Model file for the job. Use its own axes, mm. A direction names the side the tool comes from. Round coordinates to 2 decimals unless told otherwise and drop trailing zeros. Order: outer loops, then holes, each group sorted by start corner. A loop starts at its lowest first (then second) coordinate and runs counter-clockwise, first axis right, second up. Notation, with made-up numbers: (37, -31.75) -> (46, -31.75) arc R21 cw to (46, -26.75) -> close; hole circle Ø7 at (-35.75, -30.5). An arc over 180 degrees is marked (long way). Put each result on its own line as item: value. Start each with the question number.
Q1. Cut at B-B, the plane y = 91.5. List the corners of the cut face in (x, z).
Q2. Flat gauge pin, fed straight in: P1, Ø3, axis at y = 124, z = 3, coming from the +X side. Where does the tip first touch, or does it go through?
Q3. Probe L1, parallel to Y at x = 273, z = 3.9; L2, parallel to X at y = 174, z = 2.9; L3, parallel to X at y = 10, z = 4.1. List the from-to ranges inside material, lowest first.
Q4. Pull direction Y, two halves, no side cores. Call faces 1 (the face through (0, 99, 3)), 2 (the face through (25, 99, 3)), 3 (the face through (148, 0, 3)): released by +Y, released by -Y, zero draft, split by the parting line, or undercut.
Q5. 3-axis set-ups, long thin cutter, end or side, ignore diameter. For faces 4 (the face through (226, 40, 3)), 5 (the face through (115, 101, 6)), 6 (the face through (30, 99, 3)): which of +Z, -Z, +X, -X, +Y, -Y reach the whole face in a straight line?
Q6. Cut at C-C, the plane z = 3.15. State how many separate pieces and enclosed holes the cut face has, and give its area (3 significant figures).
Q7. Cut at A-A, the plane x = 217.5. List the corners of the cut face in (y, z).
from build123d import *

# Parameters (mm, degrees)
SKETCH1_W                       = 300
SKETCH1_H                       = 200
BOSS_EXTRUDE1_DEPTH             = 6
SKETCH2_W                       = 145
SKETCH2_H                       = 120
CUT_EXTRUDE1_DEPTH              = 6
SKETCH3_W                       = 5
SKETCH3_H                       = 160
CUT_EXTRUDE2_DEPTH              = 6
F_3_0MM_PRESS_DOWEL_HOLE1_D     = 3
F_3_0MM_PRESS_DOWEL_HOLE1_DEPTH = 6
F_3_0MM_PRESS_DOWEL_HOLE1_TIP   = 0.901290929


with BuildPart() as part:
    # Sketch1 → Boss-Extrude1 (new body)
    with BuildSketch(Plane.XY):
        with Locations((150, 100)):
            Rectangle(SKETCH1_W, SKETCH1_H)
    extrude(amount=BOSS_EXTRUDE1_DEPTH)

    # Sketch2 → Cut-Extrude1 (cut)
    with BuildSketch(Plane.XY):
        with Locations((227.5, 100)):
            Rectangle(SKETCH2_W, SKETCH2_H)
    extrude(amount=CUT_EXTRUDE1_DEPTH, mode=Mode.SUBTRACT)

    # Sketch3 → Cut-Extrude2 (cut)
    with BuildSketch(Plane.XY):
        with Locations((27.5, 100)):
            Rectangle(SKETCH3_W, SKETCH3_H)
    extrude(amount=CUT_EXTRUDE2_DEPTH, mode=Mode.SUBTRACT)

    # Ø3.0mm Press Dowel Hole1
    with Locations(Plane(origin=(42.474486637, -126.531359221, 6), x_dir=(1, 0, 0), z_dir=(0, 0, 1))):
        with Locations((220.525513363, 156.531359221), (102.525513363, 181.531359221), (102.525513363, 271.531359221), (89.19270005, 226.531359221), (210.525513363, 317.793651488), (230.525513363, 317.793651488), (252.525513363, 320.462332131), (232.525513363, 300.462332131), (252.525513363, 132.600386311), (232.525513363, 152.600386311), (111.286271896, 136.531359221), (91.286271896, 136.531359221), (41.525513363, 196.432813402), (13.525513363, 196.432813402), (41.525513363, 138.767959221), (13.525513363, 138.767959221), (41.525513363, 256.62990504), (13.525513363, 256.62990504), (41.525513363, 314.294759221), (13.525513363, 314.294759221)):
            Hole(F_3_0MM_PRESS_DOWEL_HOLE1_D / 2, depth=F_3_0MM_PRESS_DOWEL_HOLE1_DEPTH)
            with Locations((0, 0, -(F_3_0MM_PRESS_DOWEL_HOLE1_DEPTH + F_3_0MM_PRESS_DOWEL_HOLE1_TIP / 2))):  # 118° drill point
                Cone(0, F_3_0MM_PRESS_DOWEL_HOLE1_D / 2, F_3_0MM_PRESS_DOWEL_HOLE1_TIP, mode=Mode.SUBTRACT)


solid = part.part
Ans:
1. outline: (0, 0) -> (25, 0) -> (25, 6) -> (0, 6) -> close; (30, 0) -> (155, 0) -> (155, 6) -> (30, 6) -> close
2. P1: stops at x = 155
3. L1: y = 0 to 40, 160 to 189.76, 192.76 to 200
3. L2: x = 0 to 25, 30 to 273.5, 276.5 to 300
3. L3: x = 0 to 132.26, 135.26 to 152.26, 155.26 to 300
4. face 1: zero draft
4. face 2: undercut
4. face 3: released by -Y
5. face 4: +Z, -Z, +X
5. face 5: +Z, +X, -X, +Y, -Y
5. face 6: +Z, -Z
6. separate pieces: 1
6. enclosed holes: 21
6. area: 41,700 mm^2
7. outline: (0, 0) -> (40, 0) -> (40, 6) -> (0, 6) -> close; (160, 0) -> (200, 0) -> (200, 6) -> (160, 6) -> close
